```python
from build123d import *

# Parameters (mm, degrees)
EXTRUDE_1_DEPTH     = 6.5
CUT_EXTRUDE_2_REACH = 53.887
CUT_EXTRUDE_3_REACH = 55.094


with BuildPart() as part:
    # 草图1 → 凸台-拉伸1 (new, symmetric)
    with BuildSketch(Plane(origin=(0, 0, 0), x_dir=(0, 0, -1), z_dir=(1, 0, 0))):
        with BuildLine():
            Line((0, 0), (0, 6))
            ThreePointArc((0, 6), (5.87927664, 28.388613177), (22, 45))
            Line((22, 45), (25, 45))
            Line((25, 45), (25, 42))
            ThreePointArc((25, 42), (21.416586692, 24), (25, 6))
            Line((25, 6), (20, 6))
            Line((20, 6), (20, 0))
            Line((20, 0), (0, 0))
        make_face()
    extrude(amount=EXTRUDE_1_DEPTH, both=True)

    # 草图2 → 切除-拉伸2 (cut, up to next)
    with BuildSketch(Plane.XY, mode=Mode.PRIVATE) as cut_extrude_2_sk1:
        Polygon((-6.5, 0), (-4, 0), (-3.25, 4.253461365), (-6.5, 4.253461365), align=None)
    cut_extrude_2_tool1 = extrude(cut_extrude_2_sk1.sketch, amount=-CUT_EXTRUDE_2_REACH, mode=Mode.PRIVATE) & part.part
    # 草图2 → 切除-拉伸2 (cut, up to next)
    with BuildSketch(Plane.XY, mode=Mode.PRIVATE) as cut_extrude_2_sk2:
        Polygon((6.5, 0), (4, 0), (3.25, 4.253461365), (6.5, 4.253461365), align=None)
    cut_extrude_2_tool2 = extrude(cut_extrude_2_sk2.sketch, amount=-CUT_EXTRUDE_2_REACH, mode=Mode.PRIVATE) & part.part
    add(cut_extrude_2_tool1.solids().sort_by_distance((-5.054348, 2.219197, 0))[0], mode=Mode.SUBTRACT)
    add(cut_extrude_2_tool2.solids().sort_by_distance((5.054348, 2.219197, 0))[0], mode=Mode.SUBTRACT)

    # 草图3 → 切除-拉伸3 (cut, up to next)
    with BuildSketch(Plane(origin=(6.5, 0, 0), x_dir=(0, 0, -1), z_dir=(1, 0, 0)), mode=Mode.PRIVATE) as cut_extrude_3_sk1:
        with BuildLine():
            ThreePointArc((7.169736852, 12.07909507), (12.400276965, 12.65373917), (17.63523501, 12.120841452))
            ThreePointArc((17.63523501, 12.120841452), (19.45114939, 12.654920589), (20.008524733, 14.463820333))
            ThreePointArc((20.008524733, 14.463820333), (19.071107342, 24.389014044), (20.121422197, 34.302896243))
            ThreePointArc((20.121422197, 34.302896243), (19.130864623, 36.4613018), (16.77629627, 36.151581393))
            ThreePointArc((16.77629627, 36.151581393), (9.141463638, 26.201122888), (4.785137328, 14.439970103))
            ThreePointArc((4.785137328, 14.439970103), (5.336190032, 12.611841621), (7.169736852, 12.07909507))
        make_face()
    cut_extrude_3_tool1 = extrude(cut_extrude_3_sk1.sketch, amount=-CUT_EXTRUDE_3_REACH, mode=Mode.PRIVATE) & part.part
    add(cut_extrude_3_tool1.solids().sort_by_distance((6.5, 22.129704, -13.663141))[0], mode=Mode.SUBTRACT)


solid = part.part
```
CAD build for the part. Positions are in the model's coordinates, mm. A direction names the side the tool comes from. Round coordinates to 2 decimals unless told otherwise and drop trailing zeros. Loops run counter-clockwise (first coordinate to the right, second up) from the corner with the lowest first, then second, coordinate; pieces in that order, holes last. Notation, with made-up numbers: (24, 65.25) - (76, 65.25) arc R19 ccw to (76, 70.25) - close; hole circle Ø8 at (3, -15). An arc over 180 degrees is marked (long way). Return JSON: item names as keys, results as strings. Group by question number.
Q1. Drill centre lines: line 1 along Y through (x, z) = (4.75, -17); line 2 along Y through (x, z) = (2.5, -15.25); line 3 along Z through (x, y) = (-5.5, 19.5). Where is each one in solid material? Low to high. Write a range as [from, to].
Q2. Band-saw the part on C-C on x = 0. Give the cut face in (y, z), plus the area to 3 significant figures.
Q3. Band-saw the part on D-D on z = -4. Give the cut face in (x, y), plus the area to 3 significant figures.
Q4. Two-plate mould, pull along Z, no slides. Class faces 1 (the face through (0, 4, 0)), 2 (the face through (0.09, 26.36, -9.23)), 3 (the face through (0, 0, -10)), 4 (the face through (0.091, 12.636, -19.431)): +Z half, -Z half, draft (parallel to the pull), parting line (faces both ways), or undercut.
Q5. Flat gauge pins, fed straight in: pin 1 Ø4 at (x, z) = (-2.5, -23.5) entering from -Y; pin 2 Ø3.5 at (x, z) = (-5, -8) entering from -Y; pin 3 Ø1 at (x, z) = (5, -6) entering from -Y; pin 4 Ø3 at (x, y) = (-2.5, 4) entering from -Z. Where does each tip first touch, or does it go through?
Q6. Tool access for faces 5 (the face through (0, 6, -23)), 6 (the face through (0.09, 24.25, -19.07)), 7 (the face through (3.63, 2.1, -9.86)): list every direction of +Z, -Z, +X, -X, +Y, -Y with a clear straight run to the whole face (end or side of a thin tool).
Q7. Band-saw the part on A-A on z = -11. Give the cut face in (x, y), plus the area to 3 significant figures.
Q8. Band-saw the part on B-B on y = 29.5. Give the cut face in (x, z).
Solutions:
{
 "1": {"line 1": "y = [4.25, 12.25], [36.34, 41.5]", "line 2": "y = [0, 12.5], [34.6, 40.02]", "line 3": "z = [-21.63, -19.28], [-6.17, -2.05]"},
 "2": {"outline": "(0, -20) - (6, -20) - (6, -25) arc R47 cw to (42, -25) - (45, -25) - (45, -22) arc R45.57 ccw to (6, 0) - (0, 0) - close; hole (12.08, -7.17) arc R25 cw to (12.12, -17.64) arc R2 ccw to (14.46, -20.01) arc R50 cw to (34.3, -20.12) arc R2 ccw to (36.15, -16.78) arc R42 ccw to (14.44, -4.79) arc R2 ccw to start", "area": "506 mm^2"},
 "3": {"outline": "(-6.5, 4.25) - (-3.25, 4.25) - (-4, 0) - (4, 0) - (3.25, 4.25) - (6.5, 4.25) - (6.5, 24.67) - (-6.5, 24.67) - close", "area": "296 mm^2"},
 "4": {"face 1": "+Z half", "face 2": "undercut", "face 3": "draft", "face 4": "undercut"},
 "5": {"pin 1": "stops at y = 6", "pin 2": "stops at y = 0", "pin 3": "stops at y = 4.25", "pin 4": "stops at z = -20"},
 "6": {"face 5": "-Z, +X, -X, -Y", "face 6": "+X, -X", "face 7": "+Z, -Z, +X"},
 "7": {"outline": "(-6.5, 4.25) - (-3.25, 4.25) - (-4, 0) - (4, 0) - (3.25, 4.25) - (6.5, 4.25) - (6.5, 12.61) - (-6.5, 12.61) - close; (-6.5, 29.25) - (6.5, 29.25) - (6.5, 35.69) - (-6.5, 35.69) - close", "area": "223 mm^2"},
 "8": {"outline": "(-6.5, -21.74) - (6.5, -21.74) - (6.5, -19.36) - (-6.5, -19.36) - close; (-6.5, -11.17) - (6.5, -11.17) - (6.5, -6.53) - (-6.5, -6.53) - close"}
}
